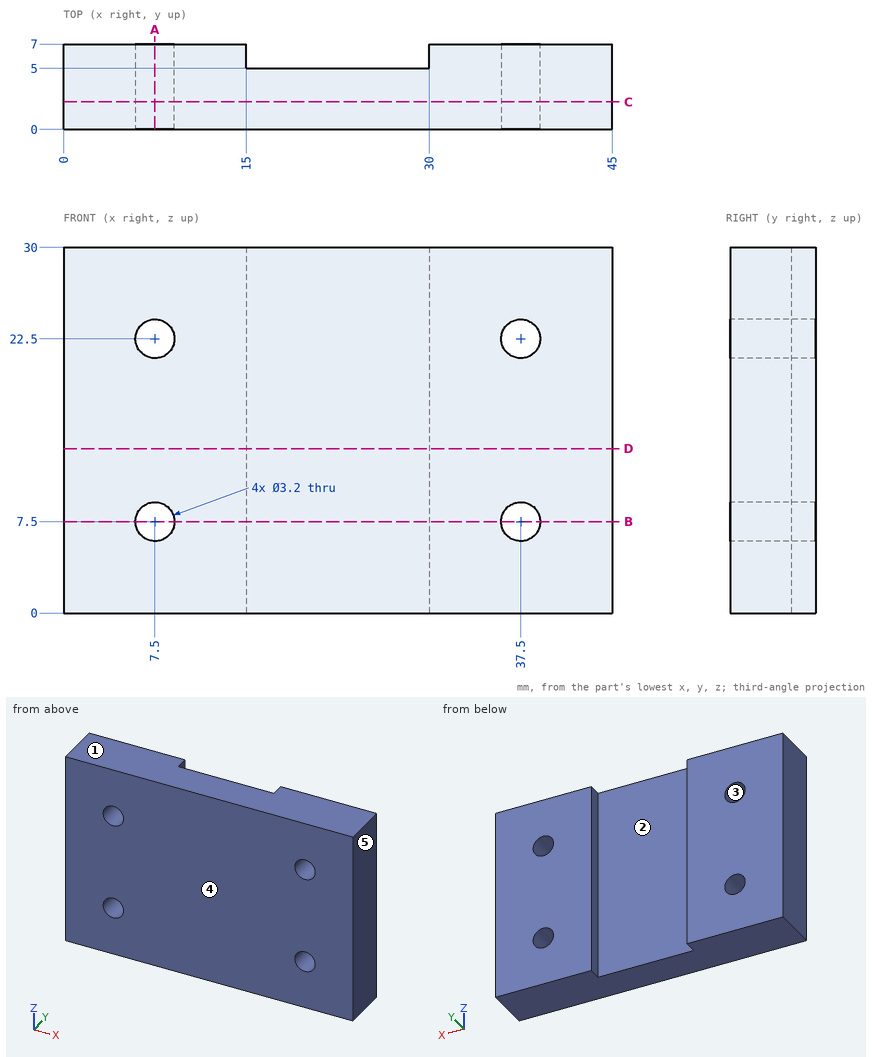
Input: dimensioned drawing with shaded views. Units: mm. Origin: part minimum x, y, z. A direction names the side the tool comes from. Give positions to 0.01 mm unless a question says otherwise; leave off trailing zeros. Loops run counter-clockwise (first coordinate to the right, second up) from the corner with the lowest first, then second, coordinate; pieces in that order, holes last. Notation, with made-up numbers: M 32,65 L 68,65 A32 cw 68,99 Z; hole C 47.5,57.25 d9. An arc over 180 degrees is marked long. Put each result on its own line as item: value.
1) Cut plane D-D, the plane z = 13.5. Return the cut outline in (x, y), plus the area to 3 significant figures.
Computed values:
outline: M 0,0 L 45,0 L 45,7 L 30,7 L 30,5 L 15,5 L 15,7 L 0,7 Z
area: 285 mm^2
2) Reachability of the marked faces 1 and 2 from +Z, -Z, +X, -X, +Y, -Y: full face, straight path, thin tool, end or side. Return the list, or none.
Computed values:
face 1: +Z, +X, -X, +Y, -Y
face 2: +Z, -Z, +Y
3) Mould query, pull axis X, two halves, no side actions, for the marked faces 3, 4 and 5. Classes: released by +X, released by -X, zero draft, split by the parting line, or undercut.
Computed values:
face 3: undercut
face 4: zero draft
face 5: released by +X
4) Material intervals for L1, parallel to X at y = 5.5, z = 22.5; L2, parallel to X at y = 2, z = 22.5; L3, parallel to X at y = 6.5, z = 20.25, sorted ascending. Write a range as from..to.
Computed values:
L1: x = 0..5.9, 9.1..15, 30..35.9, 39.1..45
L2: x = 0..5.9, 9.1..35.9, 39.1..45
L3: x = 0..15, 30..45
5) Cut plane A-A, the plane x = 7.5. Return the cut outline in (y, z).
Computed values:
outline: M 0,0 L 7,0 L 7,5.9 L 0,5.9 Z; M 0,9.1 L 7,9.1 L 7,20.9 L 0,20.9 Z; M 0,24.1 L 7,24.1 L 7,30 L 0,30 Z
6) Cut plane C-C, the plane y = 2.25. Return the cut outline in (x, z), plus the area to 3 significant figures.
Computed values:
outline: M 0,0 L 45,0 L 45,30 L 0,30 Z; hole C 7.5,7.5 d3.2; hole C 7.5,22.5 d3.2; hole C 37.5,7.5 d3.2; hole C 37.5,22.5 d3.2
area: 1,320 mm^2
7) Cut plane B-B, the plane z = 7.5. Return the cut outline in (x, y), plus the area to 3 significant figures.
Computed values:
outline: M 0,0 L 5.9,0 L 5.9,7 L 0,7 Z; M 9.1,0 L 35.9,0 L 35.9,7 L 30,7 L 30,5 L 15,5 L 15,7 L 9.1,7 Z; M 39.1,0 L 45,0 L 45,7 L 39.1,7 Z
area: 240 mm^2
8) First-contact query: P1, Ø2.5, axis at x = 37.5, z = 7.5, coming from the +Y side. Flat tip, straight axial feed; report the tip coordinate or a pass-through.
Computed values:
P1: passes through
